For this review, use the dimensioned drawing (mm, ordinates from the lowest corner) and the shaded views. A direction names the side the tool comes from. Coordinates: 2 decimals unless noted, no trailing zeros. Order: outer loops, then holes, each group sorted by start corner. A loop starts at its lowest first (then second) coordinate and runs counter-clockwise, first axis right, second up. Notation, with made-up numbers: (23.5, -28) -> (45.5, -28) arc R21 ccw to (45.5, -8) -> close; hole circle Ø1 at (-39.5, -20.5). An arc over 180 degrees is marked (long way). Return JSON: item names as keys, results as strings. Group by question number.
Item 1: Draft analysis for pull direction Z (two halves, no side actions). For the marked faces 4, 5, 6 and 7, state which applies: +Z half, -Z half, draft (parallel to the pull), parting line (faces both ways), or undercut.
Item 2: For line 1 along Z through (x, y) = (155.5, 45.5); line 2 along X through (y, z) = (12, 90); line 3 along Y through (x, z) = (52.5, 103.5), list the stretches that pass through material, from the lowest coordinate up.
Item 3: Machinability: for the marked faces 1, 2 and 3, which of the approach directions +Z, -Z, +X, -X, +Y, -Y give a long, thin tool a straight path to every point of the face, cutting with its end or side? Answer none if there is none.
Item 4: Take a section at A-A (z = 67). Write out the cut boundary in (x, y).
Item 5: Take a section at D-D (y = 21.5). Write out the cut boundary in (x, z).
Item 6: Insertion check: pin 1 (4 mm diameter, centred on y = 64, z = 59.5, fed in from +X); pin 2 (2 mm diameter, centred on y = 61, z = 87.5, fed in from -X); pin 3 (5 mm diameter, centred on x = 156.5, z = 126, fed in from -Y); pin 4 (25 mm diameter, centred on x = 102.5, z = 78, fed in from -Y). Each pin has a flat end and moves straight along its axis. Give the tip position at first contact, or say it passes through.
Item 7: Take a section at C-C (z = 126). Write out the cut boundary in (x, y), then the cut area to 3 significant figures.
Item 8: Take a section at B-B (y = 48.5). Write out the cut boundary in (x, z).
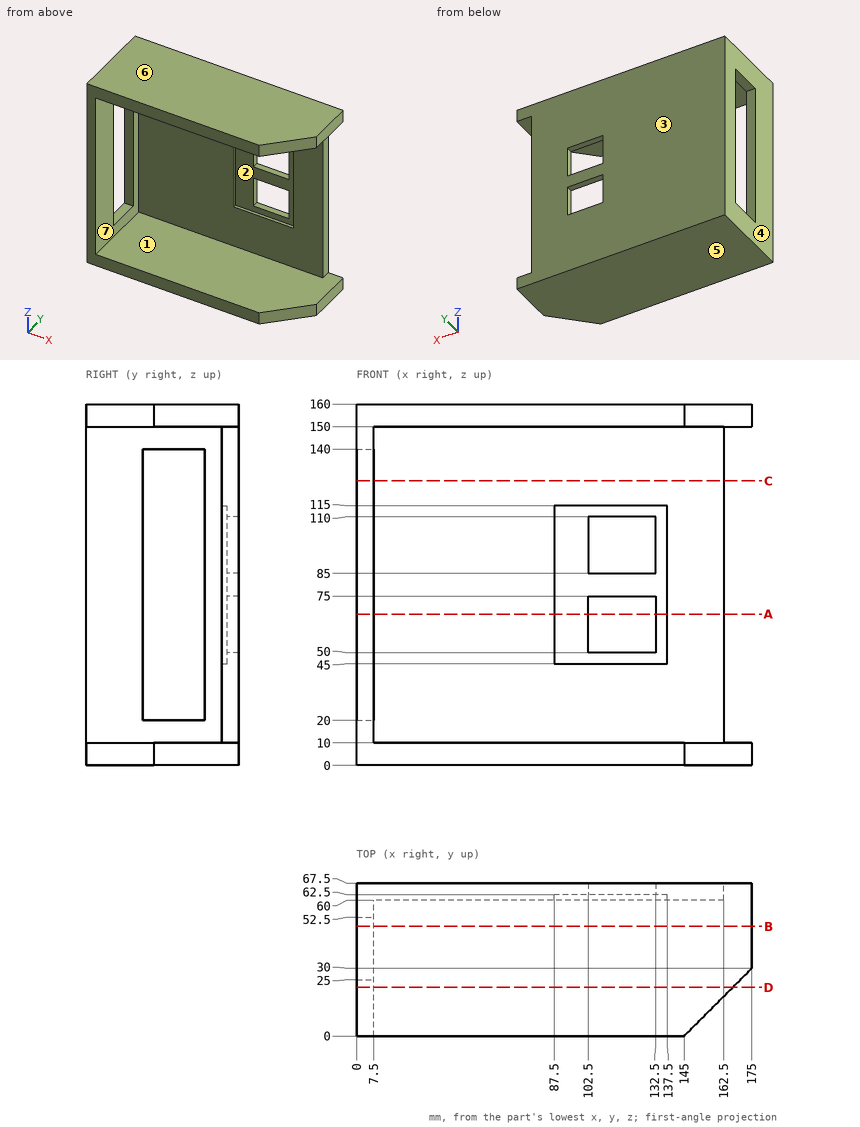
Findings below:
{
 "1": {"face 4": "draft", "face 5": "-Z half", "face 6": "+Z half", "face 7": "undercut"},
 "2": {"line 1": "z = 0 to 10, 150 to 160", "line 2": "x = 0 to 7.5", "line 3": "y = 60 to 67.5"},
 "3": {"face 1": "+X, -Y", "face 2": "-Y", "face 3": "+Z, -Z, +X, -X, +Y"},
 "4": {"outline": "(0, 0) -> (7.5, 0) -> (7.5, 25) -> (0, 25) -> close; (0, 52.5) -> (7.5, 52.5) -> (7.5, 60) -> (87.5, 60) -> (87.5, 62.5) -> (102.5, 62.5) -> (102.5, 67.5) -> (0, 67.5) -> close; (132.5, 62.5) -> (137.5, 62.5) -> (137.5, 60) -> (162.5, 60) -> (162.5, 67.5) -> (132.5, 67.5) -> close"},
 "5": {"outline": "(0, 0) -> (166.5, 0) -> (166.5, 10) -> (7.5, 10) -> (7.5, 150) -> (166.5, 150) -> (166.5, 160) -> (0, 160) -> close"},
 "6": {"pin 1": "stops at x = 162.5", "pin 2": "stops at x = 0", "pin 3": "stops at y = 60", "pin 4": "stops at y = 62.5"},
 "7": {"outline": "(0, 0) -> (7.5, 0) -> (7.5, 25) -> (0, 25) -> close; (0, 52.5) -> (7.5, 52.5) -> (7.5, 60) -> (162.5, 60) -> (162.5, 67.5) -> (0, 67.5) -> close", "area": "1,460 mm2"},
 "8": {"outline": "(0, 0) -> (175, 0) -> (175, 10) -> (7.5, 10) -> (7.5, 20) -> (0, 20) -> close; (0, 140) -> (7.5, 140) -> (7.5, 150) -> (175, 150) -> (175, 160) -> (0, 160) -> close"}
}
